Build history of the part. All positions in model axes, mm. Face numbers are marked on the shaded views. A direction names the side the tool comes from. Give positions to 0.01 mm unless a question says otherwise; leave off trailing zeros. Order: outer loops, then holes, each group sorted by start corner. A loop starts at its lowest first (then second) coordinate and runs counter-clockwise, first axis right, second up. Notation, with made-up numbers: (-27, 68) - (-14, 68) arc R30 cw to (-14, 104) - close; hole circle Ø2 at (76, 17). An arc over 180 degrees is marked (long way). Write each question's results on one line, items separated by ' | '. Start each with the question number.
1) Drill centre lines: line 1 along Y through (x, z) = (-53.5, 171.5); line 2 along X through (y, z) = (53.5, 166.5); line 3 along Z through (x, y) = (34, -38). Where is each one in solid material? Low to high. Write a range as from..to.
2) Tool access for the marked faces 3, 4, 5, 6 and 7: list every direction of +Z, -Z, +X, -X, +Y, -Y with a clear straight run to the whole face (end or side of a thin tool).
3) Drop flat-ended pins along their axis: pin 1 Ø10 at (x, y) = (39.5, -46) entering from -Z; pin 2 Ø1 at (x, y) = (15.5, 36.5) entering from +Z; pin 3 Ø4 at (x, y) = (-12, 43) entering from -Z; pin 4 Ø1.5 at (x, z) = (-10, 153.5) entering from -Y. Give the stop position or say it passes through.
4) Cut at D-D on x = -53.5. List the corners of the cut face in (y, z).
5) Cut at A-A on y = 53.5. List the corners of the cut face in (x, z), plus the area to 3 significant figures.
6) Cut at B-B on x = -16. List the corners of the cut face in (y, z).
7) Cut at C-C on z = 43. List the corners of the cut face in (x, y).
8) Two-plate mould, pull along X, no slides. Class the marked faces 1 and 2: +X half, -X half, draft (parallel to the pull), parting line (faces both ways), or undercut.
from build123d import *

# Parameters (mm, degrees)
F0_W     = 140
F0_H     = 140
F0_R     = 8.5
F0_W_2   = 120
F0_H_2   = 75
F1_DEPTH = 180
F2_W     = 20
F2_H     = 160
F2_W_2   = 100
F3_DEPTH = 140
F4_W     = 40
F4_H     = 30
F4_H_2   = 25
F5_DEPTH = 20


# Not quite as in the source:
# - a feature names something its author has since deleted; it is built from what else it names


with BuildPart() as f1:
    # F0 (on Top) → F1 (new body)
    with BuildSketch(Plane.XY):
        Rectangle(F0_W, F0_H)
        with Locations((-53.5, 53.5)):
            Circle(F0_R, mode=Mode.SUBTRACT)
        Rectangle(F0_W_2, F0_H_2, mode=Mode.SUBTRACT)
        with Locations((53.5, 53.5)):
            Circle(F0_R, mode=Mode.SUBTRACT)
    extrude(amount=F1_DEPTH)

    # F2 (on face) → F3 (cut)
    with BuildSketch(Plane.YZ.offset(70)):
        with Locations((-60, 100)):
            Rectangle(F2_W, F2_H)
        with Locations((20, 80)):
            Rectangle(F2_W_2, F2_H)
    extrude(amount=-F3_DEPTH, mode=Mode.SUBTRACT)

    # F4 (on face) → F5 (cut)
    with BuildSketch(Plane.XZ.offset(50)):
        with Locations((-30, 145)):
            Rectangle(F4_W, F4_H)
        with Locations((30, 145)):
            Rectangle(F4_W, F4_H)
        with Locations((30, 55)):
            Rectangle(F4_W, F4_H)
        with Locations((-30, 55)):
            Rectangle(F4_W, F4_H)
        with Locations((-30, 97.5)):
            Rectangle(F4_W, F4_H_2)
        with Locations((30, 97.5)):
            Rectangle(F4_W, F4_H_2)
    extrude(amount=-F5_DEPTH, mode=Mode.SUBTRACT)


solid = f1.part
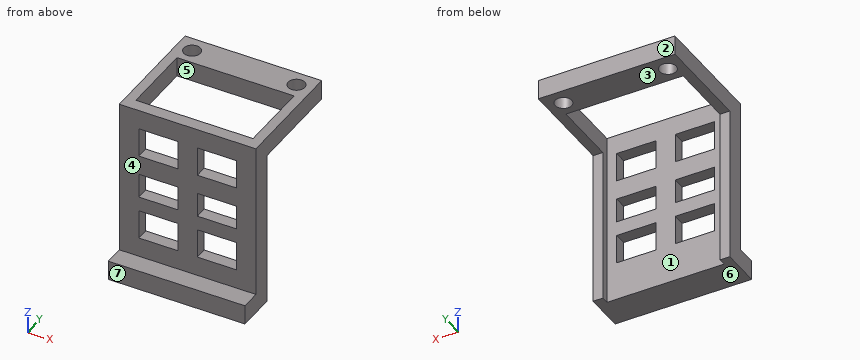
Results:
1) line 1: -50..-37.5, 37.5..45, 62..70 | line 2: -70..-62, -45..45, 62..70 | line 3: 0..40, 70..85, 110..130, 160..180
2) face 3: -Z, +X, -X, +Y | face 4: +Z, +X, -X, -Y | face 5: +Z, -Z | face 6: -Z, +X, -X, +Y, -Y | face 7: +Z, -Z, +X, -X, -Y
3) pin 1: z = 0 | pin 2: through | pin 3: z = 160 | pin 4: y = -50
4) outline: (-70, 0) - (-37.5, 0) - (-37.5, 180) - (-50, 180) - (-50, 20) - (-70, 20) - close; (37.5, 160) - (45, 160) - (45, 180) - (37.5, 180) - close; (62, 160) - (70, 160) - (70, 180) - (62, 180) - close
5) outline: (-70, 160) - (-62, 160) - (-62, 180) - (-70, 180) - close; (-45, 160) - (45, 160) - (45, 180) - (-45, 180) - close; (62, 160) - (70, 160) - (70, 180) - (62, 180) - close | area: 2,120 mm^2
6) outline: (-70, 0) - (-37.5, 0) - (-37.5, 40) - (-50, 40) - (-50, 20) - (-70, 20) - close; (-50, 70) - (-37.5, 70) - (-37.5, 85) - (-50, 85) - close; (-50, 110) - (-37.5, 110) - (-37.5, 130) - (-50, 130) - close; (-50, 160) - (-37.5, 160) - (-37.5, 180) - (-50, 180) - close; (37.5, 160) - (70, 160) - (70, 180) - (37.5, 180) - close
7) outline: (-70, -50) - (-50, -50) - (-50, -37.5) - (-60, -37.5) - (-60, -30) - (-70, -30) - close; (-10, -50) - (10, -50) - (10, -37.5) - (-10, -37.5) - close; (50, -50) - (70, -50) - (70, -30) - (60, -30) - (60, -37.5) - (50, -37.5) - close
8) face 1: undercut | face 2: draft
